```python
from build123d import *

# Parameters (mm, degrees)
SKETCH005_W             = 80
SKETCH005_H             = 20
SKETCH005_R             = 2.75
PAD010_DEPTH            = 8
POCKET009_DEPTH         = 4
SKETCH011_W             = 24.5
SKETCH011_H             = 2.666667
POCKET010_DEPTH         = 185.699521
SKETCH017_R             = 2.25
PAD011_DEPTH            = 4
BODY002_PLACEMENT_ANGLE = 180


with BuildPart() as part:
    # Sketch005 → Pad010 (new body)
    with BuildSketch(Plane.XZ):
        Rectangle(SKETCH005_W, SKETCH005_H)
        Circle(SKETCH005_R, mode=Mode.SUBTRACT)
    extrude(amount=PAD010_DEPTH)

    # Sketch007 → Pocket009 (cut)
    with BuildSketch(Plane.XZ.offset(8)):
        Polygon((4.113621, 2.375), (0, 4.75), (-4.113621, 2.375), (-4.113621, -2.375), (0, -4.75), (4.113621, -2.375), align=None)
    extrude(amount=-POCKET009_DEPTH, mode=Mode.SUBTRACT)

    # Sketch011 → Pocket010 (cut, through all)
    with BuildSketch(Plane(origin=(0, 0, 10), x_dir=(-1, 0, 0), z_dir=(0, 0, 1))):
        with Locations((-21.75, 4.333334)):
            Rectangle(SKETCH011_W, SKETCH011_H)
    pocket010 = extrude(amount=-POCKET010_DEPTH, mode=Mode.SUBTRACT)

    # Sketch017 (on Face4 of Pad010) → Pad011 (join)
    with BuildSketch(Plane(origin=(-40, 0, 0), x_dir=(0, 0, -1), z_dir=(-1, 0, 0))):
        with BuildLine():
            Line((-10, 0), (10, 0))
            Line((10, 0), (10, 41.5))
            ThreePointArc((10, 41.5), (0, 51.5), (-10, 41.5))
            Line((-10, 41.5), (-10, 0))
        make_face()
        with Locations((0, 46)):
            Circle(SKETCH017_R, mode=Mode.SUBTRACT)
    pad011 = extrude(amount=PAD011_DEPTH)

    # Mirrored007: Pad011 across YZ
    add(pad011.mirror(Plane.YZ))

    # Mirrored008: Pocket010 across YZ
    add(pocket010.mirror(Plane.YZ), mode=Mode.SUBTRACT)


with BuildPart() as part_1:
    # Body002 placement: moved
    add(part.part.moved(Location((0, 2, 9))).rotate(Axis((0, 2, 9), (1, 0, 0)), BODY002_PLACEMENT_ANGLE))


solid = part_1.part
```
The model under review builds one solid part; all positions refer to its coordinate system, in mm. A direction names the side the tool comes from. Give positions to 0.01 mm unless a question says otherwise; leave off trailing zeros. Order: outer loops, then holes, each group sorted by start corner. A loop starts at its lowest first (then second) coordinate and runs counter-clockwise, first axis right, second up. Notation, with made-up numbers: (64, 16) - (112, 16) arc R24 cw to (112, 37) - close; hole circle Ø11 at (-3.75, -0.5). An arc over 180 degrees is marked (long way). Use CSV: the item, a comma, the result in double quotes. Start each with the question number.
Q1. We need section C-C, the plane y = 22. Write out the cut boundary in (x, z).
Q2. We need section D-D, the plane z = 1. Write out the cut boundary in (x, y), and give its area (3 significant figures).
Q3. We need section A-A, the plane z = 9. State how many separate pieces and enclosed holes the cut face has, and give its area (3 significant figures).
Q4. Clearance check with flat-ended pins moving along their axes: pin 1 Ø6.5 at (x, z) = (0, 9) entering from +Y; pin 2 Ø7 at (y, z) = (48, 9) entering from +X; pin 3 Ø6 at (x, z) = (2, 12) entering from +Y. State where each tip first meets the part, or that it passes through.
Q5. Tool access review of faces 1 (the flat face through (40, 32, 9)), 2 (the flat face through (34, 6, 9)), 3 (the flat face through (-4.114, 8, 9)), 4 (the flat face through (3, 9, 19)), 5 (the cylindrical face through (42, 53.5, 9.2)): name each direction out of +Z, -Z, +X, -X, +Y, -Y from which nothing blocks a thin tool from reaching the whole face with its end or side.
Q6. The part is to be moulded in two halves that separate along Y. For faces 6 (the flat face through (-1, 2, 13)), 7 (the cylindrical face through (41.97, 50.23, 8.71)), 8 (the flat face through (22, 7.667, 9)), 9 (the flat face through (2.03, 8.03, 12.58)), say which applies: +Y half, -Y half, draft (parallel to the pull), parting line (faces both ways), or undercut.
Q7. We need section B-B, the plane x = -27. Write out the cut boundary in (y, z), and give its area (3 significant figures).
Q8. To check wall thickness, follow line 1 along Y through (x, z) = (-11.5, 15.5); line 2 along X through (y, z) = (3.1, 9); line 3 along X through (y, z) = (23.5, 12.25). State the ranges of each line that lie inside material, in increasing order. Write a range as [from, to].
Outcome:
1,outline,"(-44, -1) - (-40, -1) - (-40, 19) - (-44, 19) - close; (40, -1) - (44, -1) - (44, 19) - (40, 19) - close"
2,outline,"(-44, 2) - (44, 2) - (44, 49.5) - (40, 49.5) - (40, 10) - (-40, 10) - (-40, 49.5) - (-44, 49.5) - close; hole (-34, 5) - (-9.5, 5) - (-9.5, 7.67) - (-34, 7.67) - close; hole (9.5, 5) - (34, 5) - (34, 7.67) - (9.5, 7.67) - close"
2,area,"889 mm^2"
3,separate pieces,"4"
3,enclosed holes,"2"
3,area,"830 mm^2"
4,pin 1,"stops at y = 6"
4,pin 2,"stops at x = 44"
4,pin 3,"stops at y = 10"
5,face 1,"+Z, -Z, +Y"
5,face 2,"+Z, -Z"
5,face 3,"+Y"
5,face 4,"+Z, +X, -X, +Y, -Y"
5,face 5,"+X, -X, +Y"
6,face 6,"-Y half"
6,face 7,"undercut"
6,face 8,"undercut"
6,face 9,"draft"
7,outline,"(2, -1) - (5, -1) - (5, 19) - (2, 19) - close; (7.67, -1) - (10, -1) - (10, 19) - (7.67, 19) - close"
7,area,"107 mm^2"
8,line 1,"y = [2, 5], [7.67, 10]"
8,line 2,"x = [-44, -2.75], [2.75, 44]"
8,line 3,"x = [-44, -40], [40, 44]"
